Read the model definition and answer for the solid it produces. Units are mm, in the model's axes. A direction names the side the tool comes from. Give positions to 0.01 mm unless a question says otherwise; leave off trailing zeros. Order: outer loops, then holes, each group sorted by start corner. A loop starts at its lowest first (then second) coordinate and runs counter-clockwise, first axis right, second up.
```python
from build123d import *


with BuildPart() as f1:
    # F0 (on Top) → F1 (revolve)
    with BuildSketch(Plane.XY):
        Polygon((1.4, 6.5), (1.4, 0), (2.4, 0), (2.4, 3), (2.4, 6.5), align=None)
        Polygon((2.4, 0), (1.4, 0), (0, 0), (0, -1), (3.4, -1), (3.4, 0), (2.428727, 0), align=None)
        with BuildLine():
            Line((2.4, 3), (2.4, 0))
            Line((2.4, 0), (2.428727, 0))
            Line((2.428727, 0), (3.4, 0))
            ThreePointArc((3.4, 0), (2.746383, 1.5), (3.4, 3))
            Line((3.4, 3), (2.4, 3))
        make_face()
    revolve(axis=Axis((0, 7.587805, 0), (0, 1, 0)))


solid = f1.part
```
1) The part is cut by section D-D on y = 1.75. Determine the outline of the cut face in (x, z).
Final values:
outline: circle Ø5.52 at (0, 0); hole circle Ø2.8 at (0, 0)
2) The part is cut by section B-B on y = 3.25. Determine the outline of the cut face in (x, z), and give its area (3 significant figures).
Final values:
outline: circle Ø4.8 at (0, 0); hole circle Ø2.8 at (0, 0)
area: 11.9 mm2
3) The part is cut by section A-A on z = 0. Determine the outline of the cut face in (x, y).
Final values:
outline: (-3.4, -1) - (3.4, -1) - (3.4, 0) arc R2.05 cw to (3.4, 3) - (2.4, 3) - (2.4, 6.5) - (1.4, 6.5) - (1.4, 0) - (-1.4, 0) - (-1.4, 6.5) - (-2.4, 6.5) - (-2.4, 3) - (-3.4, 3) arc R2.05 cw to (-3.4, 0) - close
4) Given pin 1 (1.7 mm diameter, centred on x = 0, z = 0, fed in from +Y), flat-ended and moving along its own axis, determine where the tip first touches the part or whether it passes through.
Final values:
pin 1: stops at y = 0
5) Consider L1, parallel to Z at x = 0, y = 3.25; L2, parallel to X at y = 2, z = 0. Determine where each line is inside the solid, lowest interval first.
Final values:
L1: z = -2.4 to -1.4, 1.4 to 2.4
L2: x = -2.81 to -1.4, 1.4 to 2.81
6) The part is cut by section C-C on x = 0. Determine the outline of the cut face in (y, z).
Final values:
outline: (-1, -3.4) - (0, -3.4) arc R2.05 cw to (3, -3.4) - (3, -2.4) - (6.5, -2.4) - (6.5, -1.4) - (0, -1.4) - (0, 1.4) - (6.5, 1.4) - (6.5, 2.4) - (3, 2.4) - (3, 3.4) arc R2.05 cw to (0, 3.4) - (-1, 3.4) - close
7) A tool of negligible diameter and unlimited length cuts with its end or side. For faces 4 (the face through (0, -1, 0)), 5 (the face through (1.5, 3, 2.2)), from which of +Z, -Z, +X, -X, +Y, -Y can it reach the whole face along a straight path? Write none if from no direction.
Final values:
face 4: +Z, -Z, +X, -X, -Y
face 5: +Y
8) For a pull along Z with two mould halves and no side action, classify faces 1 (the face through (-0.74, -0.49, 3.32)), 2 (the face through (-1.4, 3.2, -0.06)), 3 (the face through (0, 6.5, 2)) as released by +Z, released by -Z, zero draft, split by the parting line, or undercut.
Final values:
face 1: split by the parting line
face 2: undercut
face 3: zero draft
